Check sheet for the modelled part. Datum: model origin and axes. Units: mm. A direction names the side the tool comes from. Coordinates: 2 decimals unless noted, no trailing zeros. Loops run counter-clockwise (first coordinate to the right, second up) from the corner with the lowest first, then second, coordinate; pieces in that order, holes last. Notation, with made-up numbers: M 9,89.25 L 29,89.25 A21 cw 29,120.25 Z; hole C -18.75,-27 d6. An arc over 180 degrees is marked long. Use CSV: the item, a comma, the result in double quotes. Start each with the question number.
(1) Draft check along X on faces 3 (the cylindrical face through (3.745, 3.776, -0.315)), 4 (the flat face through (1.6, 22.9, 20)), 5 (the cylindrical face through (13.32, 1.57, 15.86)). Enter one of: pulls with the +X half, pulls with the -X half, needs draft (parallel to the pull), parting line crosses it, or undercut.
(2) Section check A-A on z = 15. Record the cut outline in (x, y) (3 decimals), and give its area (3 significant figures).
(3) Section check C-C on x = 14. Record the cut outline in (y, z) (3 decimals), and give its area (3 significant figures).
(4) Set-up check for faces 1 (the flat face through (3.175, 15, 0)), 2 (the cylindrical face through (13.32, 1.57, -14.14)): record each of +Z, -Z, +X, -X, +Y, -Y from which the full face is reachable in a straight line by a thin tool's end or side.
(5) Section check D-D on z = 19.5. Record the cut outline in (x, y) (3 decimals), and give its area (3 significant figures).
(6) Scan lines: line 1 (Z direction, x = 15.4, y = 1.55); line 2 (Y direction, x = 1.95, z = -15). Record each from-to range of solid material in increasing order.
(7) Go/stop test with flat-tipped pins: pin 1 Ø5 at (y, z) = (12.5, 7.5) entering from +X (3 decimals); pin 2 Ø10 at (x, z) = (20, 5) entering from +Y (3 decimals). Record where each tip stops, or that it passes through.
(8) Section check B-B on y = 15.4. Record the cut outline in (x, z) (3 decimals), and give its area (3 significant figures).
from build123d import *

# Parameters (mm, degrees)
BOSS_EXTRUDE1_DEPTH  = 22.5
M4_CLEARANCE_HOLE1_D = 4.5
M4_CLEARANCE_HOLE2_D = 4.5
FILLET1_R            = 2
CHAMFER1_SIZE        = 5


with BuildPart() as part:
    # Sketch1 → Boss-Extrude1 (new body, symmetric)
    with BuildSketch(Plane.XY):
        Polygon((0, 0), (0, 25.4), (3.175, 25.4), (3.175, 3.175), (25.4, 3.175), (25.4, 0), align=None)
    extrude(amount=BOSS_EXTRUDE1_DEPTH, both=True)

    # M4 Clearance Hole1 (through all)
    with Locations(Plane(origin=(0, 3.175, 0), x_dir=(1, 0, 0), z_dir=(0, 1, 0))):
        with Locations((15.4, 15), (15.4, -15)):
            Hole(M4_CLEARANCE_HOLE1_D / 2)

    # M4 Clearance Hole2 (through all)
    with Locations(Plane(origin=(3.175, 0, 0), x_dir=(0, 0, -1), z_dir=(1, 0, 0))):
        with Locations((-15, 15.4), (15, 15.4)):
            Hole(M4_CLEARANCE_HOLE2_D / 2)

    # Fillet1
    fillet1_edges = [part.edges().sort_by_distance(p)[0] for p in [
        (3.175, 3.175, 0),
    ]]
    fillet(fillet1_edges, radius=FILLET1_R)

    # Chamfer1
    chamfer1_edges = [part.edges().sort_by_distance(p)[0] for p in [
        (1.5875, 25.4, 22.5),
        (1.5875, 25.4, -22.5),
        (25.4, 1.5875, -22.5),
        (25.4, 1.5875, 22.5),
    ]]
    chamfer(chamfer1_edges, length=CHAMFER1_SIZE)


solid = part.part
Outcome:
1,face 3,"pulls with the +X half"
1,face 4,"needs draft"
1,face 5,"undercut"
2,outline,"M 0,0 L 13.15,0 L 13.15,3.175 L 5.175,3.175 A2 cw 3.175,5.175 L 3.175,13.15 L 0,13.15 Z; M 0,17.65 L 3.175,17.65 L 3.175,25.4 L 0,25.4 Z; M 17.65,0 L 25.4,0 L 25.4,3.175 L 17.65,3.175 Z"
2,area,"123 mm²"
3,outline,"M 0,-22.5 L 3.175,-22.5 L 3.175,-16.761 L 0,-16.761 Z; M 0,-13.239 L 3.175,-13.239 L 3.175,13.239 L 0,13.239 Z; M 0,16.761 L 3.175,16.761 L 3.175,22.5 L 0,22.5 Z"
3,area,"121 mm²"
4,face 1,"+Z, -Z, +X, +Y"
4,face 2,"+Y, -Y"
5,outline,"M 0,0 L 23.4,0 L 23.4,3.175 L 5.175,3.175 A2 cw 3.175,5.175 L 3.175,23.4 L 0,23.4 Z"
5,area,"139 mm²"
6,line 1,"z = -22.5 to -17.25, -12.75 to 12.75, 17.25 to 22.5"
6,line 2,"y = 0 to 13.15, 17.65 to 25.4"
7,pin 1,"stops at x = 3.175"
7,pin 2,"stops at y = 3.175"
8,outline,"M 0,-22.5 L 3.175,-22.5 L 3.175,-17.25 L 0,-17.25 Z; M 0,-12.75 L 3.175,-12.75 L 3.175,12.75 L 0,12.75 Z; M 0,17.25 L 3.175,17.25 L 3.175,22.5 L 0,22.5 Z"
8,area,"114 mm²"
